Part model, mm, in its own coordinate system. Round coordinates to 2 decimals unless told otherwise and drop trailing zeros. Write each loop counter-clockwise with the first axis right and the second up, starting at its lowest first coordinate (ties: lowest second). Pieces come first, ordered by that corner, then holes. Notation, with made-up numbers: M -6.75,-14.75 L 41.25,-14.75 A29 ccw 41.25,23.25 Z; hole C -39.5,-2 d4. An arc over 180 degrees is marked long. Use one line per item in the form item = value. Start each with the question number.
Item 1: Cut at D-D, the plane x = 49. Give the cut face in (y, z).
Item 2: Probe L1, parallel to Y at x = -4, z = 1.4; L2, parallel to Y at x = 25, z = 3.7; L3, parallel to Y at x = 49, z = 0.8. List the from-to ranges inside material, lowest first.
Item 3: Cut at B-B, the plane y = 29. Give the cut face in (x, z).
Item 4: Flat gauge pins, fed straight in: pin 1 Ø6 at (x, y) = (58, 35.5) entering from -Z; pin 2 Ø1.5 at (x, z) = (10.5, 2.5) entering from +Y; pin 3 Ø2.5 at (y, z) = (93.5, 2.5) entering from -X; pin 4 Ø1.5 at (x, z) = (36.5, 2) entering from -Y. Where does each tip first touch, or does it go through?
Item 5: Cut at C-C, the plane z = 4.2. State how many separate pieces and enclosed holes the cut face has, then the cut area to 3 significant figures.
Item 6: Cut at A-A, the plane x = 82.5. Give the cut face in (y, z).
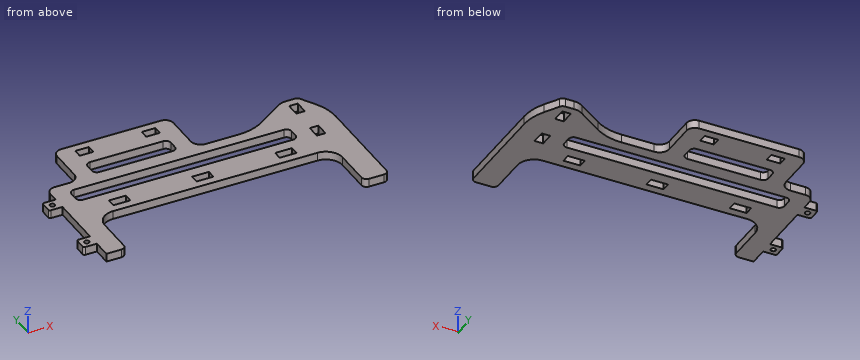
from build123d import *

# Parameters (mm, degrees)
SALIENTE_EXTRUIR1_DEPTH = 5
CROQUIS2_W              = 143
CROQUIS2_H              = 35
CORTAR_EXTRUIR1_DEPTH   = 5
REDONDEO1_R             = 10
CROQUIS3_W              = 5
CROQUIS3_H              = 8
SALIENTE_EXTRUIR2_DEPTH = 8
REDONDEO2_R             = 30
REDONDEO3_R             = 3
CROQUIS4_W              = 5.2
CROQUIS4_H              = 8.2
CORTAR_EXTRUIR2_DEPTH   = 192.034028382
REDONDEO4_R             = 3
REDONDEO5_R             = 10
REDONDEO6_R             = 1
CROQUIS5_R              = 1.5
CORTAR_EXTRUIR3_DEPTH   = 5
CROQUIS6_W              = 10.2
CROQUIS6_H              = 5.2
CORTAR_EXTRUIR4_DEPTH   = 5
CROQUIS7_W              = 132.4
CROQUIS7_H              = 10.8
CORTAR_EXTRUIR5_DEPTH   = 5
REDONDEO8_R             = 3
CROQUIS8_W              = 70
CROQUIS8_H              = 31
SALIENTE_EXTRUIR3_DEPTH = 5
CROQUIS9_W              = 8.2
CROQUIS9_H              = 5.2
CORTAR_EXTRUIR6_DEPTH   = 5
CROQUIS10_W             = 50
CROQUIS10_H             = 10.8
CORTAR_EXTRUIR7_DEPTH   = 5
REDONDEO9_R             = 3
REDONDEO10_R            = 6
REDONDEO11_R            = 5
REDONDEO12_R            = 5


with BuildPart() as part:
    # Croquis1 → Saliente-Extruir1 (new body)
    with BuildSketch(Plane.XY):
        Polygon((0, 0), (0, 70), (125, 70), (150, 87), (160, 87), (170, 70), (170, 0), align=None)
    extrude(amount=SALIENTE_EXTRUIR1_DEPTH)

    # Croquis2 → Cortar-Extruir1 (cut)
    with BuildSketch(Plane.XY.offset(5)):
        with Locations((83.5, 17.5)):
            Rectangle(CROQUIS2_W, CROQUIS2_H)
    extrude(amount=-CORTAR_EXTRUIR1_DEPTH, mode=Mode.SUBTRACT)

    # Redondeo1
    redondeo1_edges = [part.edges().sort_by_distance(p)[0] for p in [
        (12, 35, 2.5),
        (155, 35, 2.5),
    ]]
    fillet(redondeo1_edges, radius=REDONDEO1_R)

    # Croquis3 → Saliente-Extruir2 (add)
    with BuildSketch(Plane.ZY):
        with Locations((2.5, 15)):
            Rectangle(CROQUIS3_W, CROQUIS3_H)
        with Locations((2.5, 55)):
            Rectangle(CROQUIS3_W, CROQUIS3_H)
    extrude(amount=SALIENTE_EXTRUIR2_DEPTH)

    # Redondeo2
    redondeo2_edges = [part.edges().sort_by_distance(p)[0] for p in [
        (125, 70, 2.5),
        (170, 70, 2.5),
    ]]
    fillet(redondeo2_edges, radius=REDONDEO2_R)

    # Redondeo3
    redondeo3_edges = [part.edges().sort_by_distance(p)[0] for p in [
        (170, 0, 2.5),
        (12, 0, 2.5),
        (155, 0, 2.5),
    ]]
    fillet(redondeo3_edges, radius=REDONDEO3_R)

    # Croquis4 → Cortar-Extruir2 (cut, through all)
    with BuildSketch(Plane.XY.offset(5)):
        with Locations((155, 78)):
            Rectangle(CROQUIS4_W, CROQUIS4_H)
        with Locations((155, 54)):
            Rectangle(CROQUIS4_W, CROQUIS4_H)
    extrude(amount=-CORTAR_EXTRUIR2_DEPTH, mode=Mode.SUBTRACT)

    # Redondeo4
    redondeo4_edges = [part.edges().sort_by_distance(p)[0] for p in [
        (160, 87, 2.5),
    ]]
    fillet(redondeo4_edges, radius=REDONDEO4_R)

    # Redondeo5
    redondeo5_edges = [part.edges().sort_by_distance(p)[0] for p in [
        (150, 87, 2.5),
    ]]
    fillet(redondeo5_edges, radius=REDONDEO5_R)

    # Redondeo6
    redondeo6_edges = [part.edges().sort_by_distance(p)[0] for p in [
        (-8, 19, 2.5),
        (-8, 11, 2.5),
        (-8, 59, 2.5),
        (-8, 51, 2.5),
    ]]
    fillet(redondeo6_edges, radius=REDONDEO6_R)

    # Croquis5 → Cortar-Extruir3 (cut)
    with BuildSketch(Plane.XY.offset(5)):
        with Locations((-4, 55)):
            Circle(CROQUIS5_R)
        with Locations((-4, 15)):
            Circle(CROQUIS5_R)
    extrude(amount=-CORTAR_EXTRUIR3_DEPTH, mode=Mode.SUBTRACT)

    # Croquis6 → Cortar-Extruir4 (cut)
    with BuildSketch(Plane.XY.offset(5)):
        with Locations((80, 42.6)):
            Rectangle(CROQUIS6_W, CROQUIS6_H)
        with Locations((30, 42.6)):
            Rectangle(CROQUIS6_W, CROQUIS6_H)
        with Locations((130, 42.6)):
            Rectangle(CROQUIS6_W, CROQUIS6_H)
    extrude(amount=-CORTAR_EXTRUIR4_DEPTH, mode=Mode.SUBTRACT)

    # Croquis7 → Cortar-Extruir5 (cut)
    with BuildSketch(Plane.XY.offset(5)):
        with Locations((76.2, 57.6)):
            Rectangle(CROQUIS7_W, CROQUIS7_H)
    extrude(amount=-CORTAR_EXTRUIR5_DEPTH, mode=Mode.SUBTRACT)

    # Redondeo8
    redondeo8_edges = [part.edges().sort_by_distance(p)[0] for p in [
        (10, 52.2, 2.5),
        (10, 63, 2.5),
        (142.4, 63, 2.5),
        (142.4, 52.2, 2.5),
    ]]
    fillet(redondeo8_edges, radius=REDONDEO8_R)

    # Croquis8 → Saliente-Extruir3 (add)
    with BuildSketch(Plane.XY.offset(5)):
        with Locations((55, 85.5)):
            Rectangle(CROQUIS8_W, CROQUIS8_H)
    extrude(amount=-SALIENTE_EXTRUIR3_DEPTH)

    # Croquis9 → Cortar-Extruir6 (cut)
    with BuildSketch(Plane.XY.offset(5)):
        with Locations((35, 93.4)):
            Rectangle(CROQUIS9_W, CROQUIS9_H)
        with Locations((75, 93.4)):
            Rectangle(CROQUIS9_W, CROQUIS9_H)
    extrude(amount=-CORTAR_EXTRUIR6_DEPTH, mode=Mode.SUBTRACT)

    # Croquis10 → Cortar-Extruir7 (cut)
    with BuildSketch(Plane.XY.offset(5)):
        with Locations((55, 77.4)):
            Rectangle(CROQUIS10_W, CROQUIS10_H)
    extrude(amount=-CORTAR_EXTRUIR7_DEPTH, mode=Mode.SUBTRACT)

    # Redondeo9
    redondeo9_edges = [part.edges().sort_by_distance(p)[0] for p in [
        (30, 72, 2.5),
        (30, 82.8, 2.5),
        (80, 82.8, 2.5),
        (80, 72, 2.5),
    ]]
    fillet(redondeo9_edges, radius=REDONDEO9_R)

    # Redondeo10
    redondeo10_edges = [part.edges().sort_by_distance(p)[0] for p in [
        (20, 70, 2.5),
        (90, 70, 2.5),
    ]]
    fillet(redondeo10_edges, radius=REDONDEO10_R)

    # Redondeo11
    redondeo11_edges = [part.edges().sort_by_distance(p)[0] for p in [
        (20, 101, 2.5),
        (90, 101, 2.5),
    ]]
    fillet(redondeo11_edges, radius=REDONDEO11_R)

    # Redondeo12
    redondeo12_edges = [part.edges().sort_by_distance(p)[0] for p in [
        (0, 70, 2.5),
    ]]
    fillet(redondeo12_edges, radius=REDONDEO12_R)


solid = part.part
Model answer:
q1.outline = M 35,0 L 52.2,0 L 52.2,5 L 35,5 Z; M 63,0 L 72,0 L 72,5 L 63,5 Z; M 82.8,0 L 101,0 L 101,5 L 82.8,5 Z
q2.L1 = 11 to 13.5, 16.5 to 19, 51 to 53.5, 56.5 to 59
q2.L2 = 35 to 40, 45.2 to 52.2, 63 to 101
q2.L3 = 35 to 52.2, 63 to 72, 82.8 to 101
q3.outline = M 0,0 L 12.83,0 L 12.83,5 L 0,5 Z; M 154.17,0 L 170,0 L 170,5 L 154.17,5 Z
q4.pin_1 = 0
q4.pin_2 = 70
q4.pin_3 = 20
q4.pin_4 = 35
q5.separate_pieces = 1
q5.enclosed_holes = 11
q5.area = 7,400 mm²
q6.outline = M 35,0 L 40,0 L 40,5 L 35,5 Z; M 45.2,0 L 52.2,0 L 52.2,5 L 45.2,5 Z; M 63,0 L 101,0 L 101,5 L 63,5 Z
